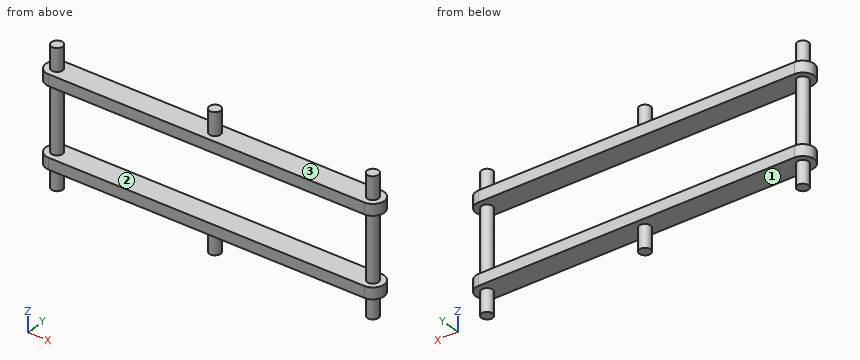
Autodesk Inventor part; units mm, degrees
ref_plane "YZ Plane" through (0, 0, 0) normal (1, 0, 0) x (0, 1, 0)
ref_plane "XZ Plane" through (0, 0, 0) normal (0, 1, 0) x (-1, 0, 0)
ref_plane "XY Plane" through (0, 0, 0) normal (0, 0, 1) x (1, 0, 0)
sketch "Sketch1" plane through (0, 0, 0) normal (0, 0, 1) x (1, 0, 0)
  line L0 (0, 0) -> (150, 0)
  line L1 (150, 0) -> (150, 10)
  line L2 (150, 10) -> (0, 10)
  line L3 (0, 10) -> (0, 0)
  dimension "d0" = 10
  dimension "d1" = 150
extrude "Extrusion1" add sketch "Sketch1" along normal blind 40
sketch "Sketch2" plane through (0, 10, 0) normal (0, 1, 0) x (1, 0, 0)
  line L0 (0, -35) -> (150, -35)
  line L1 (150, -35) -> (150, -5)
  line L2 (150, -5) -> (0, -5)
  line L3 (0, -5) -> (0, -35)
  line L4 (0, 0) -> (0, -40)
  line L5 (150, 0) -> (150, -40)
  line L6 (150, 0) -> (0, 0)
  line L7 (150, -40) -> (0, -40)
  dimension "d4" = 0
  dimension "d5" = 0
  dimension "d6" = 5
  dimension "d7" = 5
extrude "Extrusion2" cut sketch "Sketch2" against normal blind 10 contours L3 L2 L1 L0
sketch "Sketch3" plane through (0, 10, 5) normal (0, 0, 1) x (1, 0, 0)
  point P0 (0, -10)
sketch "Sketch4" plane through (0, 0, 0) normal (0, 0, -1) x (-1, 0, 0)
  circle A0 centre (-5, 5) radius 2.5
  circle A1 centre (-145, 5) radius 2.5
  line L0 (-150, 0) -> (-150, 10)
  line L1 (0, 0) -> (-150, 0)
  line L2 (-150, 10) -> (0, 10)
  line L3 (0, 10) -> (0, 0)
  circle A2 centre (-75, 5) radius 2.5
  dimension "d10" = 5
  dimension "d11" = 5
  dimension "d12" = 5
  dimension "d13" = 5
  dimension "d14" = 5
  dimension "d15" = 5
  dimension "d21" = 70
  dimension "d22" = 5
  dimension "d23" = 5
extrude "Extrusion3" add sketch "Sketch4" along normal blind 10 and the other way blind 50 contours A0 | A1
fillet "Fillet1" radius 5 8 edges at (150, 10, 37.5) (150, 10, 2.5) (0, 10, 37.5) (0, 10, 2.5) (150, 0, 37.5) (150, 0, 2.5) (0, 0, 37.5) (0, 0, 2.5)
extrude "Extrusion4" add sketch "Sketch4" along normal blind 10 contours A2
sketch "Sketch5" plane through (0, 0, 40) normal (0, 0, 1) x (1, 0, 0)
  circle A0 centre (75, 5) radius 2.5
  circle A1 centre (5, 5) radius 2.5
  line L0 (5, 0) -> (145, 0)
  point P0 (0, 0)
  dimension "d26" = 70
  dimension "d27" = 5
  dimension "d28" = 5
extrude "Extrusion5" add sketch "Sketch5" along normal blind 10 contours A0
properties part number "Joint 2"
The model under review builds one solid part; all positions refer to its coordinate system, in mm. Face numbers are marked on the shaded views. Round coordinates to 2 decimals unless told otherwise and drop trailing zeros. Loops run counter-clockwise (first coordinate to the right, second up) from the corner with the lowest first, then second, coordinate; pieces in that order, holes last.
Item 1: Take a section at A-A (x = 113). Write out the cut boundary in (y, z), then the cut area to 3 significant figures.
Determined:
outline: (0, 0) - (10, 0) - (10, 5) - (0, 5) - close; (0, 35) - (10, 35) - (10, 40) - (0, 40) - close
area: 100 mm2
Item 2: For line 1 (Z direction, x = 27, y = 8); line 2 (X direction, y = 6.75, z = -2.5); line 3 (X direction, y = 6.25, z = 27.5), list the stretches that pass through material, from the lowest coordinate up.
Determined:
line 1: z = 0 to 5, 35 to 40
line 2: x = 3.21 to 6.79, 73.21 to 76.79, 143.21 to 146.79
line 3: x = 2.83 to 7.17, 142.83 to 147.17
Item 3: Mouldability with a two-part tool opening along Z and no side actions: class the marked faces 1, 2 and 3 as released by +Z, released by -Z, zero draft, split by the parting line, or undercut.
Determined:
face 1: released by -Z
face 2: undercut
face 3: released by +Z
Item 4: Take a section at B-B (z = 20). Write out the cut boundary in (x, y).
Determined:
outline: circle Ø5 at (5, 5); circle Ø5 at (145, 5)
Item 5: Take a section at D-D (z = -4). Write out the cut boundary in (x, y), then the cut area to 3 significant figures.
Determined:
outline: circle Ø5 at (5, 5); circle Ø5 at (75, 5); circle Ø5 at (145, 5)
area: 58.9 mm2
Item 6: Take a section at C-C (x = 75). Write out the cut boundary in (y, z).
Determined:
outline: (0, 0) - (2.5, 0) - (2.5, -10) - (7.5, -10) - (7.5, 0) - (10, 0) - (10, 5) - (0, 5) - close; (0, 35) - (10, 35) - (10, 40) - (7.5, 40) - (7.5, 50) - (2.5, 50) - (2.5, 40) - (0, 40) - close
Item 7: Clearance check with flat-ended pins moving along their axes: pin 1 Ø3 at (x, y) = (99, 7) entering from -Z; pin 2 Ø3 at (x, y) = (114, 1.5) entering from +Z; pin 3 Ø1 at (y, z) = (7.5, 21.5) entering from -X. State where each tip first meets the part, or that it passes through.
Determined:
pin 1: stops at z = 0
pin 2: stops at z = 40
pin 3: stops at x = 3.5
